Check sheet for the drawn part. Datum: minimum x, y, z corner. Units: mm. Round coordinates to 2 decimals unless told otherwise and drop trailing zeros. Write each loop counter-clockwise with the first axis right and the second up, starting at its lowest first coordinate (ties: lowest second). Pieces come first, ordered by that corner, then holes. Notation, with made-up numbers: (-36.5, -19.5) - (-24.5, -19.5) arc R8 ccw to (-24.5, -10.5) - close; hole circle Ø3 at (42, 54.25). An arc over 180 degrees is marked (long way). Answer as a JSON object with one key per item and string values.
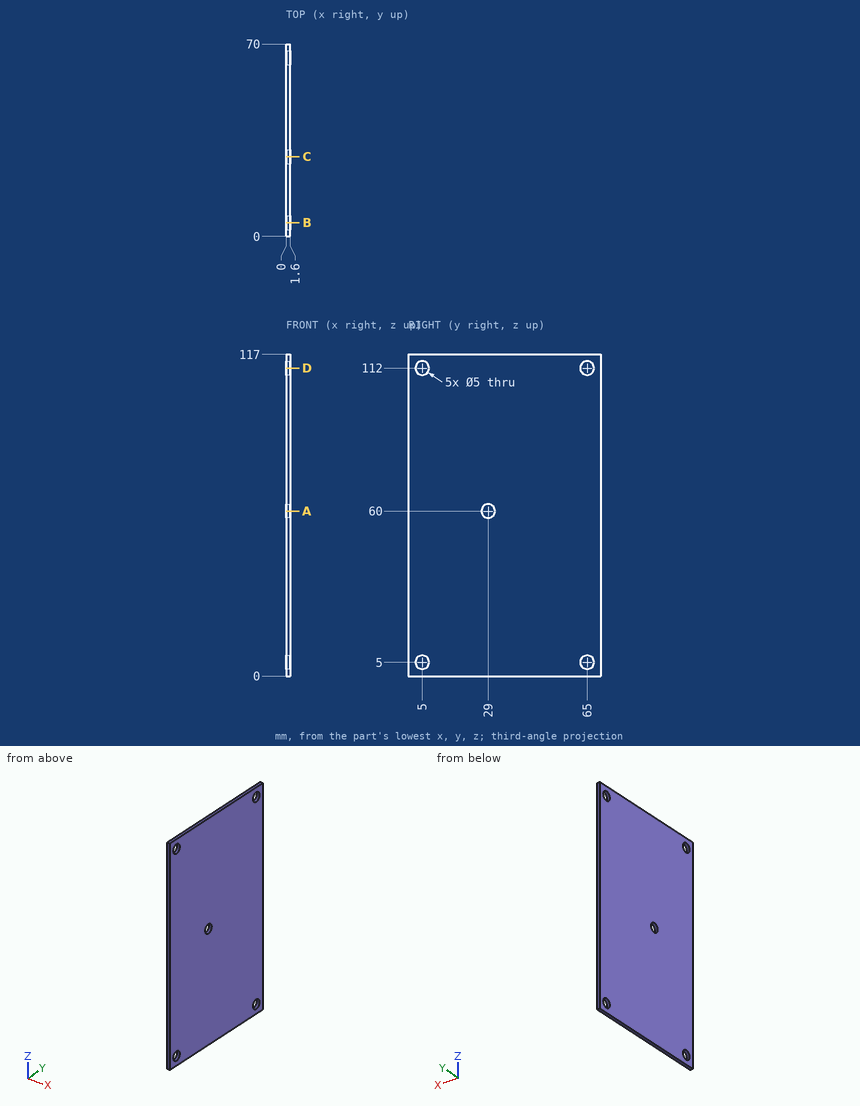
1. Cross-section at A-A (z = 60). Record the boundary of the cut face in (x, y).
Completed:
{"outline": "(0, 0) - (1.6, 0) - (1.6, 26.5) - (0, 26.5) - close; (0, 31.5) - (1.6, 31.5) - (1.6, 70) - (0, 70) - close"}
2. Material ranges on probe 1 along Y at (x, z) = (0.8, 5); probe 2 along Y at (x, z) = (0.9, 60); probe 3 along Y at (x, z) = (0.85, 59.5), recorded low to high. Write a range as from..to.
Completed:
{"probe 1": "y = 0..2.5, 7.5..62.5, 67.5..70", "probe 2": "y = 0..26.5, 31.5..70", "probe 3": "y = 0..26.55, 31.45..70"}
3. Cross-section at B-B (y = 5). Record the boundary of the cut face in (x, z).
Completed:
{"outline": "(0, 0) - (1.6, 0) - (1.6, 2.5) - (0, 2.5) - close; (0, 7.5) - (1.6, 7.5) - (1.6, 109.5) - (0, 109.5) - close; (0, 114.5) - (1.6, 114.5) - (1.6, 117) - (0, 117) - close"}
4. Cross-section at D-D (z = 112). Record the boundary of the cut face in (x, y), plus the area to 3 significant figures.
Completed:
{"outline": "(0, 0) - (1.6, 0) - (1.6, 2.5) - (0, 2.5) - close; (0, 7.5) - (1.6, 7.5) - (1.6, 62.5) - (0, 62.5) - close; (0, 67.5) - (1.6, 67.5) - (1.6, 70) - (0, 70) - close", "area": "96.0 mm^2"}
5. Cross-section at C-C (y = 29). Record the boundary of the cut face in (x, z), plus the area to 3 significant figures.
Completed:
{"outline": "(0, 0) - (1.6, 0) - (1.6, 57.5) - (0, 57.5) - close; (0, 62.5) - (1.6, 62.5) - (1.6, 117) - (0, 117) - close", "area": "179 mm^2"}
